```python
from build123d import *

# Parameters (mm, degrees)
BOSS_EXTRUDE1_DEPTH = 3.4
SKETCH3_R           = 5
CUT_EXTRUDE1_DEPTH  = 6
CUT_EXTRUDE2_DEPTH  = 10
SKETCH6_R           = 35
CUT_EXTRUDE3_DEPTH  = 10
CUT_EXTRUDE4_DEPTH  = 1
CUT_EXTRUDE5_REACH  = 87.508
SKETCH8_W           = 12
SKETCH8_H           = 35
BOSS_EXTRUDE2_DEPTH = 35
SKETCH10_R          = 4
CUT_EXTRUDE6_DEPTH  = 10


with BuildPart() as part:
    # Sketch1 → Boss-Extrude1 (new body)
    with BuildSketch(Plane.XY):
        with BuildLine():
            Line((0, -30), (80, -30))
            Line((80, -30), (80, 5))
            Line((80, 5), (48, 5))
            Line((48, 5), (16.114075804, 25.304872277))
            ThreePointArc((16.114075804, 25.304872277), (-28.802310396, 8.392074585), (0, -30))
        make_face()
    extrude(amount=BOSS_EXTRUDE1_DEPTH)

    # Sketch3 → Cut-Extrude1 (cut)
    with BuildSketch(Plane.XY.offset(3.4)):
        Circle(SKETCH3_R)
    extrude(amount=-CUT_EXTRUDE1_DEPTH, mode=Mode.SUBTRACT)

    # Sketch5 → Cut-Extrude2 (cut)
    with BuildSketch(Plane.XY.offset(3.4)):
        with BuildLine():
            ThreePointArc((0, 10), (-8.660254038, 5), (-8.660254038, -5))
            ThreePointArc((-8.660254038, -5), (-10.124355653, -10.464101615), (-15.588457268, -9))
            ThreePointArc((-15.588457268, -9), (-15.588457268, 9), (0, 18))
            ThreePointArc((0, 18), (4, 14), (0, 10))
        make_face()
    extrude(amount=-CUT_EXTRUDE2_DEPTH, mode=Mode.SUBTRACT)

    # Sketch6 → Cut-Extrude3 (cut)
    with BuildSketch(Plane(origin=(0, 0, 0), x_dir=(-1, 0, 0), z_dir=(0, 0, -1))):
        Circle(SKETCH6_R)
    extrude(amount=-CUT_EXTRUDE3_DEPTH, mode=Mode.SUBTRACT)

    # Sketch7 → Cut-Extrude4 (cut)
    with BuildSketch(Plane.XY.offset(3.4)):
        Polygon((62.77538264, -14.5), (62.77538264, -21), (64.77538264, -21), (64.77538264, -14.5), (71.27538264, -14.5), (71.27538264, -12.5), (64.77538264, -12.5), (64.77538264, -6), (62.77538264, -6), (62.77538264, -12.5), (56.27538264, -12.5), (56.27538264, -14.5), align=None)
    extrude(amount=-CUT_EXTRUDE4_DEPTH, mode=Mode.SUBTRACT)

    # Sketch8 → Cut-Extrude5 (cut, up to next)
    with BuildSketch(Plane(origin=(0, 0, 0), x_dir=(-1, 0, 0), z_dir=(0, 0, -1)), mode=Mode.PRIVATE) as cut_extrude5_sk1:
        with Locations((-74, -12.5)):
            Rectangle(SKETCH8_W, SKETCH8_H)
    cut_extrude5_tool1 = extrude(cut_extrude5_sk1.sketch, amount=-CUT_EXTRUDE5_REACH, mode=Mode.PRIVATE) & part.part
    add(cut_extrude5_tool1.solids().sort_by_distance((74, -12.5, 0))[0], mode=Mode.SUBTRACT)

    # Sketch9 → Boss-Extrude2 (add)
    with BuildSketch(Plane(origin=(0, 5, 0), x_dir=(1, 0, 0), z_dir=(0, 1, 0))):
        with BuildLine():
            Line((68, 0), (68.320508076, 0))
            ThreePointArc((68.320508076, 0), (70.908698527, 0.340741737), (73.320508076, 1.339745962))
            Line((73.320508076, 1.339745962), (77.339745962, 3.660254038))
            ThreePointArc((77.339745962, 3.660254038), (79.751555511, 4.659258263), (82.339745962, 5))
            Line((82.339745962, 5), (83, 5))
            Line((83, 5), (148, 5))
            Line((148, 5), (148, 1.6))
            Line((148, 1.6), (83, 1.6))
            Line((83, 1.6), (82.339745962, 1.6))
            ThreePointArc((82.339745962, 1.6), (80.631540264, 1.375110454), (79.039745962, 0.715767665))
            Line((79.039745962, 0.715767665), (75.020508076, -1.604740411))
            ThreePointArc((75.020508076, -1.604740411), (71.78868328, -2.943406072), (68.320508076, -3.4))
            Line((68.320508076, -3.4), (68, -3.4))
            Line((68, -3.4), (68, 0))
        make_face()
    extrude(amount=-BOSS_EXTRUDE2_DEPTH)

    # Sketch10 → Cut-Extrude6 (cut)
    with BuildSketch(Plane(origin=(0, 0, -5), x_dir=(-1, 0, 0), z_dir=(0, 0, -1))):
        with Locations((-96.339745962, -2.5)):
            Circle(SKETCH10_R)
        with Locations(Location((-96.339745962, -22.5, 0), (0, 0, 180))):
            Circle(SKETCH10_R)
    extrude(amount=-CUT_EXTRUDE6_DEPTH, mode=Mode.SUBTRACT)


solid = part.part
```
The model under review builds one solid part; all positions refer to its coordinate system, in mm. A direction names the side the tool comes from. Give positions to 0.01 mm unless a question says otherwise; leave off trailing zeros. Write each loop counter-clockwise with the first axis right and the second up, starting at its lowest first coordinate (ties: lowest second). Pieces come first, ordered by that corner, then holes. Notation, with made-up numbers: M 44,25.25 L 55,25.25 A14 ccw 55,44.25 Z; hole C 17.5,-9.5 d10. An arc over 180 degrees is marked long. Answer in a Markdown table with one row per item.
Item 1: Draft analysis for pull direction Y (two halves, no side actions). For faces 1 (the face through (39.777, 10.236, 1.676)), 2 (the face through (70.87, -12.26, -0.33)), 3 (the face through (100.155, -23.701, -3.324)), state which applies: +Y half, -Y half, draft (parallel to the pull), parting line (faces both ways), or undercut.
Check sheet entries:
| item | result |
|---|---|
| face 1 | +Y half |
| face 2 | draft |
| face 3 | undercut |
Item 2: Add section D-D on x = 108. Give the boundary of the cut face in (y, z), plus the area to 3 significant figures.
Check sheet entries:
| item | result |
|---|---|
| outline | M -30,-5 L 5,-5 L 5,-1.6 L -30,-1.6 Z |
| area | 119 mm2 |
Item 3: For line 1 along Y through (x, z) = (97, -3.5); line 2 along Y through (x, z) = (128.5, -3); line 3 along Z through (x, y) = (34, -28), list the stretches that pass through material, from the lowest coordinate up.
Check sheet entries:
| item | result |
|---|---|
| line 1 | -30 to -26.45, -18.55 to -6.45, 1.45 to 5 |
| line 2 | -30 to 5 |
| line 3 | 0 to 3.4 |
Item 4: For P1, Ø3, axis at y = -12, z = 1, coming from the -X side; P2, Ø1.1, axis at y = -13.5, z = 2.5, coming from the -X side; P3, Ø6, axis at x = 52.5, y = -0.5, coming from the -Z side; P4, Ø7, axis at x = 96.34, y = -22.5, coming from the +Z side, all flat-tipped, find the tip position at first contact; note any pin that passes through.
Check sheet entries:
| item | result |
|---|---|
| P1 | x = 32.29 |
| P2 | x = 32.06 |
| P3 | z = 0 |
| P4 | through |
Item 5: Add section A-A on x = 93.5. Give the boundary of the cut face in (y, z).
Check sheet entries:
| item | result |
|---|---|
| outline | M -30,-5 L -25.32,-5 L -25.32,-1.6 L -30,-1.6 Z; M -19.68,-5 L -5.32,-5 L -5.32,-1.6 L -19.68,-1.6 Z; M 0.32,-5 L 5,-5 L 5,-1.6 L 0.32,-1.6 Z |
Item 6: Tool access review of faces 4 (the face through (115, -12, -5)), 5 (the face through (116, -12, -1.6)), 6 (the face through (99, 5, -2)), 7 (the face through (48, -12, 0)), 8 (the face through (84, -30, -2)): name each direction out of +Z, -Z, +X, -X, +Y, -Y from which nothing blocks a thin tool from reaching the whole face with its end or side.
Check sheet entries:
| item | result |
|---|---|
| face 4 | -Z, +X, -X, +Y, -Y |
| face 5 | +Z, +X, +Y, -Y |
| face 6 | +Z, -Z, +X, +Y |
| face 7 | -Z, -X, +Y, -Y |
| face 8 | +Z, -Z, +X, -X, -Y |
Item 7: Add section C-C on y = -2.5. Give the boundary of the cut face in (x, z).
Check sheet entries:
| item | result |
|---|---|
| outline | M 34.91,0 L 68.32,0 A10 cw 73.32,-1.34 L 77.34,-3.66 A10 ccw 82.34,-5 L 92.34,-5 L 92.34,-1.6 L 82.34,-1.6 A6.6 cw 79.04,-0.72 L 75.02,1.6 A13.4 ccw 68.32,3.4 L 34.91,3.4 Z; M 100.34,-5 L 148,-5 L 148,-1.6 L 100.34,-1.6 Z |
Item 8: Add section B-B on y = -22.5. Give the boundary of the cut face in (x, z).
Check sheet entries:
| item | result |
|---|---|
| outline | M 26.81,0 L 68.32,0 A10 cw 73.32,-1.34 L 77.34,-3.66 A10 ccw 82.34,-5 L 92.34,-5 L 92.34,-1.6 L 82.34,-1.6 A6.6 cw 79.04,-0.72 L 75.02,1.6 A13.4 ccw 68.32,3.4 L 26.81,3.4 Z; M 100.34,-5 L 148,-5 L 148,-1.6 L 100.34,-1.6 Z |
